Check sheet for the modelled part. Datum: model origin and axes. Units: mm. A direction names the side the tool comes from. Give positions to 0.01 mm unless a question says otherwise; leave off trailing zeros. Order: outer loops, then holes, each group sorted by start corner. A loop starts at its lowest first (then second) coordinate and runs counter-clockwise, first axis right, second up. Notation, with made-up numbers: (-14.75, -37.75) -> (25.25, -37.75) arc R13 cw to (25.25, -30.75) -> close; hole circle Ø9 at (5.5, -8). An arc over 180 degrees is marked (long way). Answer in a Markdown table with one row per item. Add a question column.
(1) Cross-section at B-B (y = -31.2). Record the cut outline in (x, z) (3 decimals).
(2) Set-up check for faces 1 (the face through (81, -41, 2)), 2 (the face through (75.93, -40.39, 1.49)): record each of +Z, -Z, +X, -X, +Y, -Y from which the full face is reachable in a straight line by a thin tool's end or side.
(3) Cross-section at C-C (z = 1.35). State how many separate pieces and enclosed holes the cut face has, then the cut area to 3 significant figures.
(4) Go/stop test with flat-tipped pins: pin 1 (2 mm diameter, centred on x = 21, y = -55, fed in from +Z); pin 2 (0.8 mm diameter, centred on y = -39, z = 1.5, fed in from +X); pin 3 (8 mm diameter, centred on x = 68.5, y = -15.5, fed in from +Z); pin 4 (0.5 mm diameter, centred on y = -39, z = 1.5, fed in from -X). Record where each tip stops, or that it passes through.
(5) Cross-section at D-D (y = -23.5). Record the cut outline in (x, z) (3 decimals), then the cut area to 3 significant figures.
(6) Thickness scan on L1, parallel to Y at x = 81.1, z = 1.3; L2, parallel to Y at x = 31, z = 1.8; L3, parallel to Z at x = 90, y = -3.5. Record the ranges inside material, lowest first. Write a range as [from, to].
(7) Cross-section at A-A (x = 38). Record the cut outline in (y, z), then the cut area to 3 significant figures.
(8) Release check for a two-part mould opening along X. For faces 3 (the face through (-29.546, -41.224, 0.986)), 4 (the face through (35, -54, 2)) record: released by +X, released by -X, zero draft, split by the parting line, or undercut.
```python
from build123d import *

# Parameters (mm, degrees)
PAD_DEPTH    = 1
SKETCH001_R  = 5.175
PAD001_DEPTH = 1
FILLET_R     = 1


with BuildPart() as part:
    # Sketch → Pad (new body)
    with BuildSketch(Plane.XY):
        with BuildLine():
            Line((0, 0), (81.1, 0))
            ThreePointArc((60.808376, -54.9), (110.364996, -42.016654), (81.1, 0))
            Line((20.291624, -54.9), (60.808376, -54.9))
            ThreePointArc((0, 0), (-29.264996, -42.016654), (20.291624, -54.9))
        make_face()
    extrude(amount=PAD_DEPTH)

    # Sketch001 (on Face6 of Pad) → Pad001 (join)
    with BuildSketch(Plane.XY.offset(1)):
        with BuildLine():
            ThreePointArc((0, 0), (-29.264996, -42.016654), (20.291624, -54.9))
            Line((60.808376, -54.9), (20.291624, -54.9))
            ThreePointArc((60.808376, -54.9), (110.364996, -42.016654), (81.1, 0))
            Line((0, 0), (81.1, 0))
        make_face()
        with BuildLine():
            ThreePointArc((0, -2), (-27.260594, -41.664225), (19.538424, -52.9))
            Line((19.538424, -52.9), (61.561576, -52.9))
            ThreePointArc((61.561576, -52.9), (108.360594, -41.664225), (81.1, -2))
            Line((81.1, -2), (0, -2))
        make_face(mode=Mode.SUBTRACT)
        with Locations((81.1, -21.785)):
            Circle(SKETCH001_R)
        with Locations((95.425, -31.2)):
            Circle(SKETCH001_R)
        with Locations((81.1, -40.615)):
            Circle(SKETCH001_R)
        with Locations((66.775, -31.2)):
            Circle(SKETCH001_R)
        Polygon((-3.925, -19.375), (3.925, -19.375), (3.925, -27.275), (11.825, -27.275), (11.825, -35.125), (3.925, -35.125), (3.925, -43.025), (-3.925, -43.025), (-3.925, -35.125), (-11.825, -35.125), (-11.825, -27.275), (-3.925, -27.275), align=None)
    extrude(amount=PAD001_DEPTH)

    # Fillet
    fillet_edges = [part.edges().sort_by_distance(p)[0] for p in [
        (3.925, -35.125, 1.5),
        (3.925, -43.025, 1.5),
        (11.825, -35.125, 1.5),
        (11.825, -27.275, 1.5),
        (3.925, -19.375, 1.5),
        (-3.925, -43.025, 1.5),
        (-3.925, -35.125, 1.5),
        (-11.825, -35.125, 1.5),
        (-11.825, -27.275, 1.5),
        (-3.925, -27.275, 1.5),
        (-3.925, -19.375, 1.5),
        (3.925, -27.275, 1.5),
    ]]
    fillet(fillet_edges, radius=FILLET_R)


solid = part.part
```
Answer below:
| question | item | result |
|---|---|---|
| 1 | outline | (-31.2, 0) -> (112.3, 0) -> (112.3, 2) -> (110.3, 2) -> (110.3, 1) -> (100.6, 1) -> (100.6, 2) -> (90.25, 2) -> (90.25, 1) -> (71.95, 1) -> (71.95, 2) -> (61.6, 2) -> (61.6, 1) -> (11.825, 1) -> (11.825, 2) -> (-11.825, 2) -> (-11.825, 1) -> (-29.2, 1) -> (-29.2, 2) -> (-31.2, 2) -> close |
| 2 | face 1 | +Z, +X, -X, +Y, -Y |
| 2 | face 2 | +Z |
| 3 | separate pieces | 6 |
| 3 | enclosed holes | 1 |
| 3 | area | 1,360 mm² |
| 4 | pin 1 | stops at z = 2 |
| 4 | pin 2 | stops at x = 111.41 |
| 4 | pin 3 | stops at z = 1 |
| 4 | pin 4 | stops at x = -30.27 |
| 5 | outline | (-30.235, 0) -> (111.335, 0) -> (111.335, 2) -> (109.266, 2) -> (109.266, 1) -> (85.983, 1) -> (85.983, 2) -> (76.217, 2) -> (76.217, 1) -> (3.925, 1) -> (3.925, 2) -> (-3.925, 2) -> (-3.925, 1) -> (-28.166, 1) -> (-28.166, 2) -> (-30.235, 2) -> close |
| 5 | area | 163 mm² |
| 6 | L1 | y = [-62.4, -60.4], [-45.79, -35.44], [-26.96, -16.61], [-2, 0] |
| 6 | L2 | y = [-54.9, -52.9], [-2, 0] |
| 6 | L3 | z = [0, 1] |
| 7 | outline | (-54.9, 0) -> (0, 0) -> (0, 2) -> (-2, 2) -> (-2, 1) -> (-52.9, 1) -> (-52.9, 2) -> (-54.9, 2) -> close |
| 7 | area | 58.9 mm² |
| 8 | face 3 | undercut |
| 8 | face 4 | zero draft |
